```python
from build123d import *

# Parameters (mm, degrees)
SKETCH1_R           = 40
BOSS_EXTRUDE1_DEPTH = 70
SHELL1_T            = -2
SKETCH2_R           = 40
SKETCH2_R_2         = 38.8
CUT_EXTRUDE1_DEPTH  = 2
FILLET1_R           = 3


with BuildPart() as part:
    # Sketch1 → Boss-Extrude1 (new body)
    with BuildSketch(Plane(origin=(0, 0, 0), x_dir=(1, 0, 0), z_dir=(0, 1, 0))):
        with Locations(Location((0, 0, 0), (0, 0, 270))):
            Circle(SKETCH1_R)
    extrude(amount=BOSS_EXTRUDE1_DEPTH)

    # Shell1
    shell1_openings = [part.faces().sort_by_distance(p)[0] for p in [
        (0, 0, 0),
    ]]
    offset(amount=SHELL1_T, openings=shell1_openings, kind=Kind.INTERSECTION)

    # Sketch2 → Cut-Extrude1 (cut)
    with BuildSketch(Plane.XZ):
        with Locations(Location((0, 0, 0), (0, 0, 270))):
            Circle(SKETCH2_R)
        with Locations(Location((0, 0, 0), (0, 0, 270))):
            Circle(SKETCH2_R_2, mode=Mode.SUBTRACT)
    extrude(amount=-CUT_EXTRUDE1_DEPTH, mode=Mode.SUBTRACT)

    # Fillet1
    fillet1_edges = [part.edges().sort_by_distance(p)[0] for p in [
        (0, 70, -40),
    ]]
    fillet(fillet1_edges, radius=FILLET1_R)


solid = part.part
```
Design review of the part built by this model. Coordinates are the model's own, in mm. A direction names the side the tool comes from. Coordinates: 2 decimals unless noted, no trailing zeros. Order: outer loops, then holes, each group sorted by start corner. A loop starts at its lowest first (then second) coordinate and runs counter-clockwise, first axis right, second up.
1) Wall thickness on line 1 along X through (y, z) = (30, 0); line 2 along Y through (x, z) = (2.5, -25); line 3 along Z through (x, y) = (-27.5, 61.5): over which ranges is each line inside the solid? List them lowest first.
2) For faces 1 (the flat face through (-25.7, 0, 28.6)), 2 (the flat face through (1, 68, -1)), list the 3-axis set-ups (+Z, -Z, +X, -X, +Y, -Y) from which the entire face can be reached by the end or side of a thin tool; tool diameter is ignored.
3) Take a section at A-A, the plane z = 0. Give the boundary of the cut face in (x, y).
4) Take a section at C-C, the plane x = 0. Give the boundary of the cut face in (y, z).
5) Mouldability with a two-part tool opening along X and no side actions: class faces 3 (the cylindrical face through (-23.122, 33.524, -30.156)), 4 (the cylindrical face through (11.65, 0.99, -37.01)), 5 (the flat face through (21, 2, 33)) as +X half, -X half, draft (parallel to the pull), parting line (faces both ways), or undercut.
6) Clearance check with flat-ended pins moving along their axes: pin 1 (4 mm diameter, centred on x = 22, z = 12.5, fed in from -Y); pin 2 (1.5 mm diameter, centred on y = 27, z = -12.5, fed in from +X); pin 3 (2 mm diameter, centred on x = -24.5, y = 57.5, fed in from -Z). State where each tip first meets the part, or that it passes through.
7) Take a section at B-B, the plane y = 65. Give the boundary of the cut face in (x, z).
Returned:
1. line 1: x = -40 to -38, 38 to 40
1. line 2: y = 68 to 70
1. line 3: z = -29.05 to -26.22, 26.22 to 29.05
2. face 1: +Z, -Z, +X, -X, -Y
2. face 2: -Y
3. outline: (-40, 2) - (-38.8, 2) - (-38.8, 0) - (-38, 0) - (-38, 68) - (38, 68) - (38, 0) - (38.8, 0) - (38.8, 2) - (40, 2) - (40, 67) arc R3 ccw to (37, 70) - (-37, 70) arc R3 ccw to (-40, 67) - close
4. outline: (0, -38.8) - (2, -38.8) - (2, -40) - (67, -40) arc R3 ccw to (70, -37) - (70, 37) arc R3 ccw to (67, 40) - (2, 40) - (2, 38.8) - (0, 38.8) - (0, 38) - (68, 38) - (68, -38) - (0, -38) - close
5. face 3: undercut
5. face 4: parting line
5. face 5: draft
6. pin 1: stops at y = 68
6. pin 2: stops at x = 38.24
6. pin 3: stops at z = -32.37
7. outline: circle Ø80 at (0, 0); hole circle Ø76 at (0, 0)
